from build123d import *

# Parameters (mm, degrees)
BOSS_EXTRUDE1_DEPTH = 20
SKETCH3_R           = 4.1
CUT_EXTRUDE1_DEPTH  = 77.978565174
SKETCH4_R           = 4.1
CUT_EXTRUDE2_DEPTH  = 69.374877828
FILLET1_R           = 7


with BuildPart() as part:
    # Sketch1 → Boss-Extrude1 (new body)
    with BuildSketch(Plane(origin=(0, 0, 0), x_dir=(1, 0, 0), z_dir=(0, 1, 0))):
        Polygon((-22.986013986, 8.601398601), (-22.986013986, -11.398601399), (-5.986013986, -11.398601399), (-5.986013986, -2.307692308), (8.013986014, -2.307692308), (8.013986014, -11.398601399), (25.013986014, -11.398601399), (25.013986014, 8.601398601), (6.013986014, 8.601398601), (6.013986014, 58.601398601), (-3.986013986, 58.601398601), (-3.986013986, 8.601398601), align=None)
    extrude(amount=BOSS_EXTRUDE1_DEPTH)

    # Sketch3 → Cut-Extrude1 (cut, through all)
    with BuildSketch(Plane.XY.offset(11.398601399)):
        with Locations((-14.486013986, 10)):
            Circle(SKETCH3_R)
        with Locations((16.513986014, 10)):
            Circle(SKETCH3_R)
    extrude(amount=-CUT_EXTRUDE1_DEPTH, mode=Mode.SUBTRACT)

    # Sketch4 → Cut-Extrude2 (cut, through all)
    with BuildSketch(Plane(origin=(6.013986014, 0, 0), x_dir=(0, 0, -1), z_dir=(1, 0, 0))):
        with Locations((28.601398601, 10)):
            Circle(SKETCH4_R)
        with Locations((48.601398601, 10)):
            Circle(SKETCH4_R)
    extrude(amount=-CUT_EXTRUDE2_DEPTH, mode=Mode.SUBTRACT)

    # Fillet1
    fillet1_edges = [part.edges().sort_by_distance(p)[0] for p in [
        (-5.986013986, 10, 2.307692308),
        (8.013986014, 10, 2.307692308),
    ]]
    fillet(fillet1_edges, radius=FILLET1_R - 0.0001)  # a hair under: the kernel refuses the full size


solid = part.part
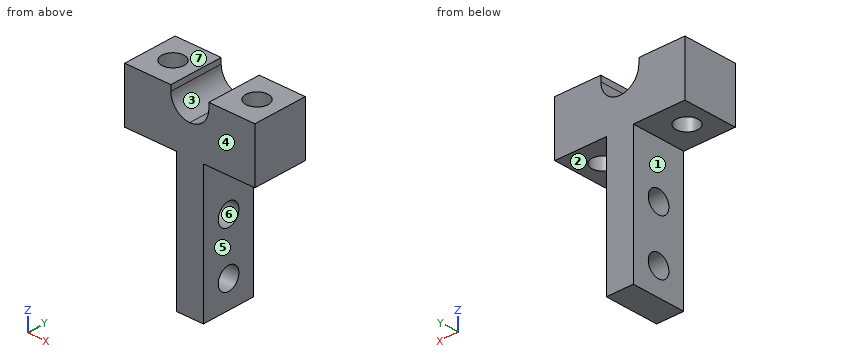
Design review of the part built by this model. Coordinates are the model's own, in mm. Face numbers are marked on the shaded views. A direction names the side the tool comes from. Give positions to 0.01 mm unless a question says otherwise; leave off trailing zeros. Loops run counter-clockwise (first coordinate to the right, second up) from the corner with the lowest first, then second, coordinate; pieces in that order, holes last. Notation, with made-up numbers: M 71,75.25 L 78,75.25 A21 ccw 78,87.25 Z; hole C 15.25,-33.75 d5. An arc over 180 degrees is marked long. Answer as a JSON object with one key per item and string values.
Item 1: We need section B-B (z = 7.5). State the section outline as (x, y) points, and give its area (3 significant figures).
Output values:
{"outline": "M -22.99,0 L -5.75,0 L -5.75,20 L -22.99,20 Z; M 7.78,0 L 25.01,0 L 25.01,20 L 7.78,20 Z; hole C -14.49,10 d8.2; hole C 16.51,10 d8.2", "area": "584 mm2"}
Item 2: We need section A-A (y = 10). Count the separate pieces of the cut face and the enclosed holes in it, and give its area (3 significant figures).
Output values:
{"separate pieces": "5", "enclosed holes": "0", "area": "862 mm2"}
Item 3: For P1, Ø8, axis at y = 9, z = -25, coming from the -X side; P2, Ø10, axis at y = 6.5, z = -33, coming from the +X side; P3, Ø9.5, axis at x = -14.5, y = 12, coming from the -Z side, all flat-tipped, find the tip position at first contact; note any pin that passes through.
Output values:
{"P1": "stops at x = -3.99", "P2": "stops at x = 6.01", "P3": "stops at z = -8.6"}
Item 4: Wall thickness on line 1 along X through (y, z) = (2, 9); line 2 along Z through (x, y) = (5, 13.5); line 3 along Z through (x, y) = (-1.5, 13.75): over which ranges is each line inside the solid? List them lowest first.
Output values:
{"line 1": "x = -22.99 to -5.98, 8.01 to 25.01", "line 2": "z = -58.6 to -50.74, -46.47 to -30.74, -26.47 to 3.55", "line 3": "z = -58.6 to -50.26, -46.94 to -30.26, -26.94 to 2.77"}
Item 5: Machinability: for the marked faces 1, 2, 3 and 4, which of the approach directions +Z, -Z, +X, -X, +Y, -Y give a long, thin tool a straight path to every point of the face, cutting with its end or side? Answer none if there is none.
Output values:
{"face 1": "-Z, -X, +Y, -Y", "face 2": "-Z, +X, +Y, -Y", "face 3": "+Z, +Y, -Y", "face 4": "+Z, -Z, +X, -X, -Y"}
Item 6: Mouldability with a two-part tool opening along Z and no side actions: class the marked faces 5, 6 and 7 as pulls with the +Z half, pulls with the -Z half, needs draft (parallel to the pull), parting line crosses it, or undercut.
Output values:
{"face 5": "needs draft", "face 6": "undercut", "face 7": "pulls with the +Z half"}
Item 7: We need section C-C (x = 15). State the section outline as (y, z) points.
Output values:
{"outline": "M 0,-8.6 L 6.19,-8.6 L 6.19,11.4 L 0,11.4 Z; M 13.81,-8.6 L 20,-8.6 L 20,11.4 L 13.81,11.4 Z"}
